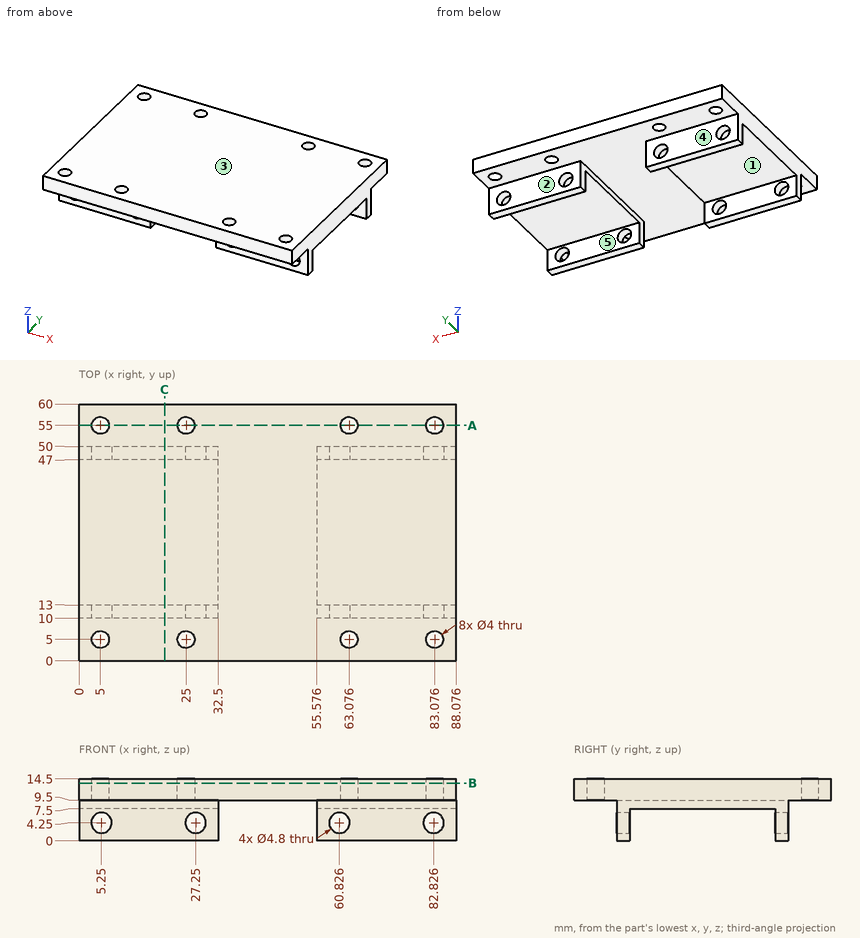
Drawing for the job (mm, zero at the part's lowest x, y, z). A direction names the side the tool comes from. Give positions to 0.01 mm unless a question says otherwise; leave off trailing zeros. Loops run counter-clockwise (first coordinate to the right, second up) from the corner with the lowest first, then second, coordinate; pieces in that order, holes last.
(1) Pull direction Y, two halves, no side cores. Call the marked faces 3, 4 and 5: pulls with the +Y half, pulls with the -Y half, needs draft (parallel to the pull), parting line crosses it, or undercut.
Return value:
face 3: needs draft
face 4: pulls with the +Y half
face 5: undercut
(2) Band-saw the part on C-C (x = 20). Write the cut outline in (y, z), and give its area (3 significant figures).
Return value:
outline: (0, 9.5) - (10, 9.5) - (10, 0) - (13, 0) - (13, 7.5) - (47, 7.5) - (47, 0) - (50, 0) - (50, 9.5) - (60, 9.5) - (60, 14.5) - (0, 14.5) - close
area: 425 mm2
(3) 3-axis set-ups, long thin cutter, end or side, ignore diameter. For the marked faces 1 and 2: which of +Z, -Z, +X, -X, +Y, -Y reach the whole face in a straight line?
Return value:
face 1: -Z, +X, -X
face 2: -Z, +X, -X, +Y
(4) Band-saw the part on B-B (z = 13.5). Count the separate pieces of the cut face and the enclosed holes in it, and give its area (3 significant figures).
Return value:
separate pieces: 1
enclosed holes: 8
area: 5,180 mm2
(5) Band-saw the part on A-A (y = 55). Write the cut outline in (x, z).
Return value:
outline: (0, 9.5) - (3, 9.5) - (3, 14.5) - (0, 14.5) - close; (7, 9.5) - (23, 9.5) - (23, 14.5) - (7, 14.5) - close; (27, 9.5) - (61.08, 9.5) - (61.08, 14.5) - (27, 14.5) - close; (65.08, 9.5) - (81.08, 9.5) - (81.08, 14.5) - (65.08, 14.5) - close; (85.08, 9.5) - (88.08, 9.5) - (88.08, 14.5) - (85.08, 14.5) - close
(6) Pin check, flat tips, straight feed: pin 1 (6.5 mm diameter, centred on x = 63.08, y = 5, fed in from +Z); pin 2 (6 mm diameter, centred on x = 73, y = 26.5, fed in from -Z); pin 3 (7.5 mm diameter, centred on x = 65.5, z = 4.5, fed in from +Y); pin 4 (4.5 mm diameter, centred on x = 5, y = 5, fed in from -Z). Stop position of each tip, or through.
Return value:
pin 1: stops at z = 14.5
pin 2: stops at z = 7.5
pin 3: stops at y = 50
pin 4: stops at z = 9.5
(7) Drill centre lines: line 1 along X through (y, z) = (11.1, 4.25); line 2 along Y through (x, z) = (22.5, 1); line 3 along X through (y, z) = (14.5, 9.25). Where is each one in solid material? Low to high.
Return value:
line 1: x = 0 to 2.85, 7.65 to 24.85, 29.65 to 32.5, 55.58 to 58.43, 63.23 to 80.43, 85.23 to 88.08
line 2: y = 10 to 13, 47 to 50
line 3: x = 0 to 32.5, 55.58 to 88.08
